from build123d import *

# Parameters (mm, degrees)
F2_DEPTH = 1250
F1_R     = 6.5
F3_DEPTH = 25


with BuildPart() as f2:
    # F1 (on Top) → F2 (new body)
    with BuildSketch(Plane.XY):
        with BuildLine():
            Line((-80, 80), (-80, -80))
            Line((-80, -80), (-67, -80))
            Line((-67, -80), (-67, -19))
            ThreePointArc((-67, -19), (-62.6066017178, -8.3933982822), (-52, -4))
            Line((-52, -4), (52, -4))
            ThreePointArc((52, -4), (62.6066017178, -8.3933982822), (67, -19))
            Line((67, -19), (67, -80))
            Line((67, -80), (80, -80))
            Line((80, -80), (80, 80))
            Line((80, 80), (67, 80))
            Line((67, 80), (67, 19))
            ThreePointArc((67, 19), (62.6066017178, 8.3933982822), (52, 4))
            Line((52, 4), (-52, 4))
            ThreePointArc((-52, 4), (-62.6066017178, 8.3933982822), (-67, 19))
            Line((-67, 19), (-67, 80))
            Line((-67, 80), (-80, 80))
        make_face()
    extrude(amount=-F2_DEPTH)

    # F1 (on Top) → F3 (join)
    with BuildSketch(Plane.XY):
        with BuildLine():
            Line((67, 80), (-67, 80))
            Line((-67, 80), (-67, 19))
            ThreePointArc((-67, 19), (-62.6066017178, 8.3933982822), (-52, 4))
            Line((-52, 4), (52, 4))
            ThreePointArc((52, 4), (62.6066017178, 8.3933982822), (67, 19))
            Line((67, 19), (67, 80))
        make_face()
        with Locations((-47.5, 60.5)):
            Circle(F1_R, mode=Mode.SUBTRACT)
        with Locations((47.5, 60.5)):
            Circle(F1_R, mode=Mode.SUBTRACT)
        with BuildLine():
            Line((-80, 80), (-80, -80))
            Line((-80, -80), (-67, -80))
            Line((-67, -80), (-67, -19))
            ThreePointArc((-67, -19), (-62.6066017178, -8.3933982822), (-52, -4))
            Line((-52, -4), (52, -4))
            ThreePointArc((52, -4), (62.6066017178, -8.3933982822), (67, -19))
            Line((67, -19), (67, -80))
            Line((67, -80), (80, -80))
            Line((80, -80), (80, 80))
            Line((80, 80), (67, 80))
            Line((67, 80), (67, 19))
            ThreePointArc((67, 19), (62.6066017178, 8.3933982822), (52, 4))
            Line((52, 4), (-52, 4))
            ThreePointArc((-52, 4), (-62.6066017178, 8.3933982822), (-67, 19))
            Line((-67, 19), (-67, 80))
            Line((-67, 80), (-80, 80))
        make_face()
        with BuildLine():
            Line((-67, -19), (-67, -80))
            Line((-67, -80), (67, -80))
            Line((67, -80), (67, -19))
            ThreePointArc((67, -19), (62.6066017178, -8.3933982822), (52, -4))
            Line((52, -4), (-52, -4))
            ThreePointArc((-52, -4), (-62.6066017178, -8.3933982822), (-67, -19))
        make_face()
        with Locations((-47.5, -60.5)):
            Circle(F1_R, mode=Mode.SUBTRACT)
        with Locations((47.5, -60.5)):
            Circle(F1_R, mode=Mode.SUBTRACT)
    extrude(amount=-F3_DEPTH)

    # F4: F2 across face


with BuildPart() as f2_1:
    add(f2.part)
    add(f2.part.mirror(Plane(origin=(0, 0, -1250), x_dir=(1, 0, 0), z_dir=(0, 0, -1))))


solid = f2_1.part
Model file for the job. Use its own axes, mm. A direction names the side the tool comes from. Coordinates: 2 decimals unless noted, no trailing zeros. Write each loop counter-clockwise with the first axis right and the second up, starting at its lowest first coordinate (ties: lowest second). Pieces come first, ordered by that corner, then holes. Notation, with made-up numbers: (-29, -8.75) - (21, -8.75) arc R27 ccw to (21, 14.25) - close; hole circle Ø5 at (37.5, -27.5). An arc over 180 degrees is marked (long way). Write each question's results on one line, items separated by ' | '. Start each with the question number.
1) Cut at B-B (x = 17.5). Write the cut outline in (y, z), then the cut area to 3 significant figures.
2) Mould opens along X. For faces 1 (the face through (1, 4, -1267)), 2 (the face through (80, -1, -1268)), 3 (the face through (-1, 1, -2500)) say: pulls with the +X half, pulls with the -X half, needs draft (parallel to the pull), parting line crosses it, or undercut.
3) Flat gauge pins, fed straight in: P1, Ø11.5, axis at x = -47.5, y = 60.5, coming from the +Z side; P2, Ø5, axis at x = -61.5, z = -529.5, coming from the +Y side; P3, Ø6, axis at x = -53, z = -1769.5, coming from the +Y side; P4, Ø10, axis at x = 54.5, z = -280.5, coming from the -Y side. Where does each tip first touch, or does it go through?
4) 3-axis set-ups, long thin cutter, end or side, ignore diameter. For faces 4 (the face through (-1, 43, -25)), 5 (the face through (-80, 1, -1268)), 6 (the face through (-1, -4, -1267)): which of +Z, -Z, +X, -X, +Y, -Y reach the whole face in a straight line?
5) Probe line 1 along X through (y, z) = (60, -13); line 2 along Y through (x, z) = (47.5, -11.25); line 3 along Z through (x, y) = (53, 37.5). List the from-to ranges inside material, lowest first. Write a range as from..to.
6) Cut at A-A (z = -1028.5). Write the cut outline in (x, y).
Returned:
1) outline: (-80, -2500) - (80, -2500) - (80, -2475) - (4, -2475) - (4, -25) - (80, -25) - (80, 0) - (-80, 0) - (-80, -25) - (-4, -25) - (-4, -2475) - (-80, -2475) - close | area: 27,600 mm^2
2) face 1: undercut | face 2: pulls with the +X half | face 3: needs draft
3) P1: through | P2: y = 10 | P3: y = 4.54 | P4: y = -6.01
4) face 4: +Y | face 5: +Z, -Z, -X, +Y, -Y | face 6: -Y
5) line 1: -80..-53.98, -41.02..41.02, 53.98..80 | line 2: -80..-67, -54..54, 67..80 | line 3: -2500..-2475, -25..0
6) outline: (-80, -80) - (-67, -80) - (-67, -19) arc R15 cw to (-52, -4) - (52, -4) arc R15 cw to (67, -19) - (67, -80) - (80, -80) - (80, 80) - (67, 80) - (67, 19) arc R15 cw to (52, 4) - (-52, 4) arc R15 cw to (-67, 19) - (-67, 80) - (-80, 80) - close
